from build123d import *

# Parameters (mm, degrees)
SKETCH1_W           = 31.75
SKETCH1_H           = 9.525
BOSS_EXTRUDE1_DEPTH = 3
SKETCH2_R           = 1.5875
CUT_EXTRUDE1_DEPTH  = 17.843308204
FILLET1_R           = 4.572
SKETCH3_W           = 9.525
SKETCH3_H           = 3
BOSS_EXTRUDE2_DEPTH = 6
BOSS_EXTRUDE3_DEPTH = 9.525
FILLET3_R           = 2.54
FILLET4_R           = 1
FILLET5_R           = 2.54
FILLET7_R           = 1


with BuildPart() as part:
    # Sketch1 → Boss-Extrude1 (new body)
    with BuildSketch(Plane(origin=(0, 0, 0), x_dir=(1, 0, 0), z_dir=(0, 1, 0))):
        Rectangle(SKETCH1_W, SKETCH1_H)
    extrude(amount=BOSS_EXTRUDE1_DEPTH)

    # Sketch2 → Cut-Extrude1 (cut, through all)
    with BuildSketch(Plane(origin=(0, 3, 0), x_dir=(1, 0, 0), z_dir=(0, 1, 0))):
        with Locations(Location((-9.525, 0, 0), (0, 0, 270))):
            Circle(SKETCH2_R)
        with Locations(Location((9.525, 0, 0), (0, 0, 270))):
            Circle(SKETCH2_R)
    extrude(amount=-CUT_EXTRUDE1_DEPTH, mode=Mode.SUBTRACT)

    # Fillet1
    fillet1_edges = [part.edges().sort_by_distance(p)[0] for p in [
        (-15.875, 1.5, 4.7625),
        (-15.875, 1.5, -4.7625),
    ]]
    fillet(fillet1_edges, radius=FILLET1_R)

    # Sketch3 → Boss-Extrude2 (add)
    with BuildSketch(Plane(origin=(15.875, 0, 0), x_dir=(0, 0, -1), z_dir=(1, 0, 0))):
        with Locations((0, 1.5)):
            Rectangle(SKETCH3_W, SKETCH3_H)
    extrude(amount=BOSS_EXTRUDE2_DEPTH)

    # Sketch5 → Boss-Extrude3 (add)
    with BuildSketch(Plane.XY.offset(4.7625)):
        Polygon((18.875, 3), (18.875, 14.451976797), (24.524350343, 19.794466274), (26.718222037, 19.794466274), (26.718222037, 16.794466274), (25.718222037, 16.794466274), (21.875, 13.16), (21.875, 3), align=None)
    extrude(amount=-BOSS_EXTRUDE3_DEPTH)

    # Fillet3
    # the kernel refuses this fillet: 2.54 mm, written as the material it adds along each edge
    with BuildSketch(Plane(origin=(21.875, 13.16, 4.7625), x_dir=(0, -1, 0), z_dir=(0, 0, -1))) as fillet3_piece_1:
        with BuildLine():
            CenterArc((FILLET3_R * 0.430658932297, -FILLET3_R), FILLET3_R, 90, 46.599119654)
            Line((-FILLET3_R * 0.295905181539, -FILLET3_R * 0.312901325509), (0, 0))
            Line((0, 0), (FILLET3_R * 0.430658932297, 0))
        make_face()
    extrude(amount=9.525)
    with BuildSketch(Plane(origin=(25.718222037, 16.794466274, 4.7625), x_dir=(-0.7265641138352414, -0.6870986744906513, 0), z_dir=(0, 0, -1))) as fillet3_piece_2_section:
        with BuildLine():
            CenterArc((FILLET3_R * 0.39795723135, -FILLET3_R), FILLET3_R, 90, 43.400880346)
            Line((-FILLET3_R * 0.28914144314, -FILLET3_R * 0.273435886165), (0, 0))
            Line((0, 0), (FILLET3_R * 0.39795723135, 0))
        make_face()
    fillet3_piece_2 = extrude(amount=9.525, mode=Mode.PRIVATE)
    fillet3_piece_2 = split(fillet3_piece_2, bisect_by=Plane(origin=(26.718222037, 16.648240502, 0), z_dir=(-1, 0, 0)), keep=Keep.TOP, mode=Mode.PRIVATE)
    add(fillet3_piece_2)

    # Fillet4
    fillet4_edges = [part.edges().sort_by_distance(p)[0] for p in [
        (18.875, 14.451976797, 0),
        (24.524350343, 19.794466274, 0),
        (26.718222037, 19.794466274, 0),
        (26.718222037, 16.794443265, 0),
    ]]
    fillet(fillet4_edges, radius=FILLET4_R)

    # Fillet5
    fillet5_edges = [part.edges().sort_by_distance(p)[0] for p in [
        (18.875, 3, 0),
    ]]
    fillet(fillet5_edges, radius=FILLET5_R)

    # Fillet7
    fillet7_edges = [part.edges().sort_by_distance(p)[0] for p in [
        (18.875, 9.780658932, -4.7625),
        (2.516, 3, -4.7625),
        (18.131051224, 3.743948776, 4.7625),
        (18.131051224, 3.743948776, -4.7625),
        (2.516, 3, 4.7625),
        (-15.875, 3, 0),
        (-14.535892204, 3, -3.423392204),
        (-14.535892204, 3, 3.423392204),
        (21.875, 6.033063156, -4.7625),
        (21.875, 6.033063156, 4.7625),
        (23.826786069, 15.005769142, -4.7625),
        (23.826786069, 15.005769142, 4.7625),
        (22.082138473, 13.070793966, 4.7625),
        (22.082138473, 13.070793966, -4.7625),
        (25.459186859, 16.454259389, 4.7625),
        (21.711555113, 17.134456183, -4.7625),
        (21.711555113, 17.134456183, 4.7625),
        (26.718222037, 18.220775531, 4.7625),
        (25.320264806, 19.794466274, 4.7625),
        (18.875, 9.780658932, 4.7625),
        (26.519951397, 17.049397551, 4.7625),
        (26.425328818, 19.501573055, 4.7625),
        (24.552553679, 19.723596005, 4.7625),
        (18.95655058, 14.416856311, 4.7625),
        (25.320264806, 19.794466274, -4.7625),
        (26.718222037, 18.220775531, -4.7625),
        (25.459186859, 16.454259389, -4.7625),
        (26.519951397, 17.049397551, -4.7625),
        (26.425328818, 19.501573055, -4.7625),
        (24.552553679, 19.723596005, -4.7625),
        (18.95655058, 14.416856311, -4.7625),
    ]]
    fillet(fillet7_edges, radius=FILLET7_R)


solid = part.part
Model file for the job. Use its own axes, mm. A direction names the side the tool comes from. Coordinates: 2 decimals unless noted, no trailing zeros. Write each loop counter-clockwise with the first axis right and the second up, starting at its lowest first coordinate (ties: lowest second). Pieces come first, ordered by that corner, then holes. Notation, with made-up numbers: (-14.75, 65.5) - (41.25, 65.5) arc R12 cw to (41.25, 85.5) - close; hole circle Ø4 at (-9.5, -0.75). An arc over 180 degrees is marked (long way). Write each question's results on one line, items separated by ' | '. Start each with the question number.
1) Probe line 1 along X through (y, z) = (0.9, 0) (1 decimal); line 2 along Y through (x, z) = (12.5, -1); line 3 along X through (y, z) = (2.3, 0) (1 decimal). List the from-to ranges inside material, lowest first. Write a range as from..to.
2) Cut at B-B (y = 1.5). Count the separate pieces of the cut face and the enclosed holes in it, then the cut area to 3 significant figures.
3) Mould opens along X. For faces 5 (the face through (21.59, 5.95, -4.46)), 6 (the face through (18.151, 3.764, -0.053)), 7 (the face through (7.975, 1.521, -0.344)), 8 (the face through (8.1, 1.8, 4.762)) say: pulls with the +X half, pulls with the -X half, needs draft (parallel to the pull), parting line crosses it, or undercut.
4) 3-axis set-ups, long thin cutter, end or side, ignore diameter. For faces 1 (the face through (2.323, 2.715, 4.462)), 2 (the face through (2.709, 2.715, -4.462)), 3 (the face through (18.875, 10, 0)), 4 (the face through (21.875, 6, 0)): which of +Z, -Z, +X, -X, +Y, -Y reach the whole face in a straight line?
5) Flat gauge pins, fed straight in: P1, Ø4, axis at x = -5, z = 0.5, coming from the +Y side; P2, Ø5, axis at x = 21.5, z = -1, coming from the +Y side. Where does each tip first touch, or does it go through?
6) Cut at C-C (x = -1). Write the cut outline in (y, z), then the cut area to 3 significant figures.
7) Cut at A-A (y = 7.75). Write the cut outline in (x, z) (1 decimal), then the cut area to 3 significant figures.
Returned:
1) line 1: -15.9..-11.1, -7.9..7.9, 11.1..21.9 | line 2: 0..3 | line 3: -15.8..-11.1, -7.9..7.9, 11.1..21.9
2) separate pieces: 1 | enclosed holes: 2 | area: 334 mm^2
3) face 5: pulls with the +X half | face 6: pulls with the -X half | face 7: undercut | face 8: needs draft
4) face 1: +Z, -X, +Y | face 2: -Z, -X, +Y | face 3: +Z, -Z, -X, +Y | face 4: +Z, -Z, +X, -Y
5) P1: y = 3 | P2: y = 19.3
6) outline: (0, -4.76) - (2, -4.76) arc R1 ccw to (3, -3.76) - (3, 3.76) arc R1 ccw to (2, 4.76) - (0, 4.76) - close | area: 28.1 mm^2
7) outline: (18.9, -3.8) arc R1 ccw to (19.9, -4.8) - (20.9, -4.8) arc R1 ccw to (21.9, -3.8) - (21.9, 3.8) arc R1 ccw to (20.9, 4.8) - (19.9, 4.8) arc R1 ccw to (18.9, 3.8) - close | area: 27.7 mm^2
